Autodesk Inventor part; units mm, degrees
ref_plane "YZ Plane" through (0, 0, 0) normal (1, 0, 0) x (0, 1, 0)
ref_plane "XZ Plane" through (0, 0, 0) normal (0, 1, 0) x (-1, 0, 0)
ref_plane "XY Plane" through (0, 0, 0) normal (0, 0, 1) x (1, 0, 0)
sketch "Skizze1" plane through (0, 0, 0) normal (1, 0, 0) x (0, 1, 0)
  line L0 (-14.5799, 0) -> (14.5799, 0)
  line L1 (0, -14.5799) -> (0, 14.5799)
  line L2 (9.5, 3) -> (9.5, 3.5)
  line L3 (9.5, 3.5) -> (10, 3.5)
  line L4 (8.5, 3) -> (8.5, 6.2861)
  line L5 (7.7861, 6.2861) -> (4.5, 3)
  line L6 (8.5, 6.2861) -> (7.7861, 6.2861)
  line L7 (8.5, 3) -> (9.5, 3)
  line L8 (9.5, -3) -> (9.5, -3.5)
  line L9 (9.5, -3.5) -> (10, -3.5)
  line L10 (8.5, -3) -> (8.5, -6.2861)
  line L11 (7.7861, -6.2861) -> (4.5, -3)
  line L12 (8.5, -6.2861) -> (7.7861, -6.2861)
  line L13 (8.5, -3) -> (9.5, -3)
  line L14 (10, 3.5) -> (10, 8)
  line L15 (10, -3.5) -> (10, -8)
  line L16 (-9.5, 3) -> (-9.5, 3.5)
  line L17 (-9.5, 3.5) -> (-10, 3.5)
  line L18 (-8.5, 3) -> (-8.5, 6.2861)
  line L19 (-7.7861, 6.2861) -> (-4.5, 3)
  line L20 (-8.5, 6.2861) -> (-7.7861, 6.2861)
  line L21 (-8.5, 3) -> (-9.5, 3)
  line L22 (-8.5, -3) -> (-9.5, -3)
  line L23 (-8.5, -3) -> (-8.5, -6.2861)
  line L24 (-8.5, -6.2861) -> (-7.7861, -6.2861)
  line L25 (-7.7861, -6.2861) -> (-4.5, -3)
  line L26 (-9.5, -3) -> (-9.5, -3.5)
  line L27 (-9.5, -3.5) -> (-10, -3.5)
  line L28 (3, -9.5) -> (3.5, -9.5)
  line L29 (3.5, -9.5) -> (3.5, -10)
  line L30 (3, -8.5) -> (6.2861, -8.5)
  line L31 (6.2861, -7.7861) -> (3, -4.5)
  line L32 (6.2861, -8.5) -> (6.2861, -7.7861)
  line L33 (3, -8.5) -> (3, -9.5)
  line L34 (-3, -8.5) -> (-3, -9.5)
  line L35 (-3, -8.5) -> (-6.2861, -8.5)
  line L36 (-6.2861, -8.5) -> (-6.2861, -7.7861)
  line L37 (-6.2861, -7.7861) -> (-3, -4.5)
  line L38 (-3, -9.5) -> (-3.5, -9.5)
  line L39 (-3.5, -9.5) -> (-3.5, -10)
  line L40 (3.5, 9.5) -> (3.5, 10)
  line L41 (3, 9.5) -> (3.5, 9.5)
  line L42 (3, 8.5) -> (3, 9.5)
  line L43 (3, 8.5) -> (6.2861, 8.5)
  line L44 (6.2861, 8.5) -> (6.2861, 7.7861)
  line L45 (6.2861, 7.7861) -> (3, 4.5)
  line L46 (-6.2861, 7.7861) -> (-3, 4.5)
  line L47 (-6.2861, 8.5) -> (-6.2861, 7.7861)
  line L48 (-3, 8.5) -> (-6.2861, 8.5)
  line L49 (-3, 8.5) -> (-3, 9.5)
  line L50 (-3, 9.5) -> (-3.5, 9.5)
  line L51 (-3.5, 9.5) -> (-3.5, 10)
  line L52 (8, 10) -> (3.5, 10)
  line L53 (-3.5, 10) -> (-8, 10)
  line L54 (-10, 8) -> (-10, 3.5)
  line L55 (-10, -3.5) -> (-10, -8)
  line L56 (-8, -10) -> (-3.5, -10)
  line L57 (3.5, -10) -> (8, -10)
  arc A0 (10, 8) -> (8, 10) centre (8, 8) ccw
  arc A1 (8, -10) -> (10, -8) centre (8, -8) ccw
  arc A2 (-10, -8) -> (-8, -10) centre (-8, -8) ccw
  arc A3 (-8, 10) -> (-10, 8) centre (-8, 8) ccw
  line L58 (-2.8201, 2.0744) -> (-2.113, 2.7815)
  line L59 (-2.113, 2.7815) -> (-1.5814, 2.2498)
  line L60 (-2.2813, 1.5356) -> (-2.8201, 2.0744)
  line L61 (2.8201, 2.0744) -> (2.113, 2.7815)
  line L62 (2.113, 2.7815) -> (1.5814, 2.2498)
  line L63 (2.2813, 1.5356) -> (2.8201, 2.0744)
  line L64 (2.0744, -2.8201) -> (2.7815, -2.113)
  line L65 (2.7815, -2.113) -> (2.2498, -1.5814)
  line L66 (1.5356, -2.2813) -> (2.0744, -2.8201)
  line L67 (-2.7815, -2.113) -> (-2.2498, -1.5814)
  line L68 (-2.0744, -2.8201) -> (-2.7815, -2.113)
  line L69 (-1.5356, -2.2813) -> (-2.0744, -2.8201)
  arc A4 (1.5814, 2.2498) -> (-1.5814, 2.2498) centre (0, 0) ccw
  arc A5 (1.5814, 2.2498) -> (-1.5814, 2.2498) centre (0, 0) ccw
  arc A6 (2.2498, -1.5814) -> (2.2813, 1.5356) centre (0, 0) ccw
  arc A7 (2.2498, -1.5814) -> (2.2813, 1.5356) centre (0, 0) ccw
  arc A8 (-2.2813, 1.5356) -> (-2.2498, -1.5814) centre (0, 0) ccw
  arc A9 (-1.5356, -2.2813) -> (1.5356, -2.2813) centre (0, 0) ccw
  arc A10 (-2.2813, 1.5356) -> (-2.2498, -1.5814) centre (0, 0) ccw
  arc A11 (-1.5356, -2.2813) -> (1.5356, -2.2813) centre (0, 0) ccw
  line L70 (0.3484, 4.5) -> (-0.0051, 4.1465)
  line L71 (-0.0051, 4.1465) -> (-0.3589, 4.5)
  line L72 (3, 4.5) -> (0.3484, 4.5)
  line L73 (-0.3589, 4.5) -> (-3, 4.5)
  line L74 (4.5, 0.3484) -> (4.1465, -0.0051)
  line L75 (4.1465, -0.0051) -> (4.5, -0.3589)
  line L76 (0.3484, -4.5) -> (-0.0051, -4.1465)
  line L77 (-0.0051, -4.1465) -> (-0.3589, -4.5)
  line L78 (-4.5, 0.3484) -> (-4.1465, -0.0051)
  line L79 (-4.1465, -0.0051) -> (-4.5, -0.3589)
  line L80 (4.5, 3) -> (4.5, 0.3484)
  line L81 (4.5, -0.3589) -> (4.5, -3)
  line L82 (3, -4.5) -> (0.3484, -4.5)
  line L83 (-0.3589, -4.5) -> (-3, -4.5)
  line L84 (-4.5, 3) -> (-4.5, 0.3484)
  line L85 (-4.5, -0.3589) -> (-4.5, -3)
  point P0 (-10, -10)
  point P1 (-10, 10)
  point P2 (10, -10)
  dimension "d0" = 20
  dimension "d1" = 20
  dimension "d4" = 6
  dimension "d9" = 0.5
  dimension "d10" = 0.5
  dimension "d13" = 45
  dimension "d14" = 3.2861
  dimension "d16" = 3
  dimension "d17" = 3.5
  dimension "d19" = 6
  dimension "d20" = 0.5
  dimension "d21" = 0.5
  dimension "d22" = 45
  dimension "d23" = 3.2861
  dimension "d25" = 2
extrude "Extrusion1" add sketch "Skizze1" along normal mid plane 120 contours L78 L84 L19 L20 L18 L21 L16 L17 L54 A3 L53 L51 L50 L49 L48 L47 L46 L73 L71 L70 L1 A4 L59 L58 L60 A8 L0 | L0 A8 L67 L68 L69 A9 L1 L76 L77 L83 L37 L36 L35 L34 L38 L39 L56 A2 L55 L27 L26 L22 L23 L24 L25 L85 L79 L78 | A6 L63 L61 L62 A4 L1 L70 L72 L45 L44 L43 L42 L41 L40 L52 A0 L14 L3 L2 L7 L4 L6 L5 L80 L74 L0 | L0 L74 L75 L81 L11 L12 L10 L13 L8 L9 L15 A1 L57 L29 L28 L33 L30 L32 L31 L82 L76 L1 A9 L66 L64 L65 A6
properties part number "Motedius_20x20_B-Type_Slot-6_120" material "Aluminium 6061"
Input: part model. Units: mm. Frame: model coordinates. A direction names the side the tool comes from. Coordinates: 2 decimals unless noted, no trailing zeros.
Q1. Contact query for flat-ended pins moving along their axis: pin 1 (0.5 mm diameter, centred on x = 17.5, z = 9, fed in from +Y); pin 2 (4 mm diameter, centred on x = -28.5, y = -0.5, fed in from -Z); pin 3 (1.5 mm diameter, centred on x = 5.5, z = 0.5, fed in from +Y). Output: stop coordinate, or through.
Q2. Set-up query: faces 1 (the face through (-1, 5, 8.5)), 2 (the face through (-1, -2, 4.5)), 3 (the face through (-1, 4.5, -2)), 4 (the face through (-1, -4.5, -2)), 5 (the face through (-1, -2, -4.5)). Return all of +Z, -Z, +X, -X, +Y, -Y with unobstructed straight access to the full face (end or side cutting, diameter ignored); none if empty.
Q3. Material intervals for line 1 (Y direction, x = -54, z = 8); line 2 (Z direction, x = -30.5, y = 4.25); line 3 (Z direction, x = 36, y = 0), sorted ascending.
Working result:
1. pin 1: stops at y = 9.85
1. pin 2: stops at z = -4.5
1. pin 3: stops at y = 4.5
2. face 1: +X, -X
2. face 2: +Z, +X, -X
2. face 3: +X, -X, +Y
2. face 4: +X, -X, -Y
2. face 5: -Z, +X, -X
3. line 1: y = -10 to -6.29, 6.29 to 10
3. line 2: z = -10 to -8.5, -5.75 to -0.11, 0.1 to 5.75, 8.5 to 10
3. line 3: z = -4.15 to -2.75, 2.75 to 4.15
